from build123d import *

# Parameters (mm, degrees)
BASE_FLANGE1_DEPTH         = 1
SKETCHED_START             = 31
SKETCHED_BEND1_DEPTH       = 178
SKETCHED_BEND1_2_DEPTH     = 128
SKETCHED_BEND1_3_DEPTH     = 178
SKETCHED_BEND1_4_OUTLINE_W = 128
SKETCHED_BEND1_4_OUTLINE_H = 1
SKETCHED_BEND1_4_DEPTH     = 29.234623369
SKETCHED_START_2           = 210.765376631
SKETCHED_BEND1_5_OUTLINE_W = 128
SKETCHED_BEND1_5_OUTLINE_H = 1
SKETCHED_BEND1_5_DEPTH     = 29.234623369
SKETCHED_BEND1_6_DEPTH     = 128
SKETCHED_BEND1_7_OUTLINE_W = 178
SKETCHED_BEND1_7_OUTLINE_H = 1
SKETCHED_BEND1_7_DEPTH     = 29.234623369
SKETCHED_START_3           = 160.765376631
SKETCHED_BEND1_8_OUTLINE_W = 178
SKETCHED_BEND1_8_OUTLINE_H = 1
SKETCHED_BEND1_8_DEPTH     = 29.234623369


# Read off the part's stored shape, not the designer's step: Sketched Bend1
# Sheet-metal steps are written as plain solids
with BuildPart() as part:
    # Sketch1 → Base-Flange1 (new body)
    with BuildSketch(Plane.XY):
        Polygon((0, 209), (31, 209), (31, 240), (159, 240), (159, 209), (190, 209), (190, 31), (159, 31), (159, 0), (31, 0), (31, 31), (0, 31), align=None)
    extrude(amount=-BASE_FLANGE1_DEPTH)

    # Sketched Bend1 outline → Sketched Bend1 (add)
    with BuildSketch(Plane(origin=(0, 0, 0), x_dir=(1, 0, 0), z_dir=(0, 1, 0)).offset(SKETCHED_START)):
        with BuildLine():
            Line((29.234623369, -0.7366), (29.234623369, -29.765376631))
            Line((29.234623369, -29.765376631), (30.234623369, -29.765376631))
            Line((30.234623369, -29.765376631), (30.234623369, -0.7366))
            ThreePointArc((30.234623369, -0.7366), (30.450368514, -0.215745145), (30.971223369, 0))
            Line((30.971223369, 0), (29.398582279, 0))
            ThreePointArc((29.398582279, 0), (29.276108612, -0.359286442), (29.234623369, -0.7366))
        make_face()
        with BuildLine():
            Line((160.601417721, 0), (159.028776631, 0))
            ThreePointArc((159.028776631, 0), (159.549631486, -0.215745145), (159.765376631, -0.7366))
            Line((159.765376631, -0.7366), (159.765376631, -29.765376631))
            Line((159.765376631, -29.765376631), (160.765376631, -29.765376631))
            Line((160.765376631, -29.765376631), (160.765376631, -0.7366))
            ThreePointArc((160.765376631, -0.7366), (160.723891388, -0.359286442), (160.601417721, 0))
        make_face()
    extrude(amount=SKETCHED_BEND1_DEPTH)

    # Sketched Bend1 2 outline → Sketched Bend1 2 (add)
    with BuildSketch(Plane.YZ.offset(SKETCHED_START)):
        with BuildLine():
            Line((209.028776631, 0), (210.601417721, 0))
            ThreePointArc((210.601417721, 0), (210.723891388, 0.359286442), (210.765376631, 0.7366))
            Line((210.765376631, 0.7366), (210.765376631, 29.765376631))
            Line((210.765376631, 29.765376631), (209.765376631, 29.765376631))
            Line((209.765376631, 29.765376631), (209.765376631, 0.7366))
            ThreePointArc((209.765376631, 0.7366), (209.549631486, 0.215745145), (209.028776631, 0))
        make_face()
        with BuildLine():
            ThreePointArc((29.234623369, 0.7366), (29.276108612, 0.359286442), (29.398582279, 0))
            Line((29.398582279, 0), (30.971223369, 0))
            ThreePointArc((30.971223369, 0), (30.450368514, 0.215745145), (30.234623369, 0.7366))
            Line((30.234623369, 0.7366), (30.234623369, 29.765376631))
            Line((30.234623369, 29.765376631), (29.234623369, 29.765376631))
            Line((29.234623369, 29.765376631), (29.234623369, 0.7366))
        make_face()
    extrude(amount=SKETCHED_BEND1_2_DEPTH)

    # Sketched Bend1 3 outline → Sketched Bend1 3 (cut)
    with BuildSketch(Plane(origin=(0, 0, 0), x_dir=(1, 0, 0), z_dir=(0, 1, 0)).offset(SKETCHED_START)):
        with BuildLine():
            Line((0, 0), (29.398582279, 0))
            ThreePointArc((29.398582279, 0), (30.039397205, 0.728828115), (30.971223369, 1))
            Line((30.971223369, 1), (0, 1))
            Line((0, 1), (0, 0))
        make_face()
        with BuildLine():
            Line((190, 1), (159.028776631, 1))
            ThreePointArc((159.028776631, 1), (159.960602795, 0.728828115), (160.601417721, 0))
            Line((160.601417721, 0), (190, 0))
            Line((190, 0), (190, 1))
        make_face()
    extrude(amount=SKETCHED_BEND1_3_DEPTH, mode=Mode.SUBTRACT)

    # Sketched Bend1 4 outline → Sketched Bend1 4 (cut)
    with BuildSketch(Plane(origin=(0, 0, 0), x_dir=(1, 0, 0), z_dir=(0, 1, 0))):
        with Locations((95, 0.5)):
            Rectangle(SKETCHED_BEND1_4_OUTLINE_W, SKETCHED_BEND1_4_OUTLINE_H)
    extrude(amount=SKETCHED_BEND1_4_DEPTH, mode=Mode.SUBTRACT)

    # Sketched Bend1 5 outline → Sketched Bend1 5 (cut)
    with BuildSketch(Plane(origin=(0, 0, 0), x_dir=(1, 0, 0), z_dir=(0, 1, 0)).offset(SKETCHED_START_2)):
        with Locations((95, 0.5)):
            Rectangle(SKETCHED_BEND1_5_OUTLINE_W, SKETCHED_BEND1_5_OUTLINE_H)
    extrude(amount=SKETCHED_BEND1_5_DEPTH, mode=Mode.SUBTRACT)

    # Sketched Bend1 6 outline → Sketched Bend1 6 (cut)
    with BuildSketch(Plane.YZ.offset(SKETCHED_START)):
        with BuildLine():
            ThreePointArc((210.601417721, 0), (209.960602795, -0.728828115), (209.028776631, -1))
            Line((209.028776631, -1), (240, -1))
            Line((240, -1), (240, 0))
            Line((240, 0), (210.601417721, 0))
        make_face()
        with BuildLine():
            Line((0, -1), (30.971223369, -1))
            ThreePointArc((30.971223369, -1), (30.039397205, -0.728828115), (29.398582279, 0))
            Line((29.398582279, 0), (0, 0))
            Line((0, 0), (0, -1))
        make_face()
    extrude(amount=SKETCHED_BEND1_6_DEPTH, mode=Mode.SUBTRACT)

    # Sketched Bend1 7 outline → Sketched Bend1 7 (cut)
    with BuildSketch(Plane.YZ):
        with Locations((120, -0.5)):
            Rectangle(SKETCHED_BEND1_7_OUTLINE_W, SKETCHED_BEND1_7_OUTLINE_H)
    extrude(amount=SKETCHED_BEND1_7_DEPTH, mode=Mode.SUBTRACT)

    # Sketched Bend1 8 outline → Sketched Bend1 8 (cut)
    with BuildSketch(Plane.YZ.offset(SKETCHED_START_3)):
        with Locations((120, -0.5)):
            Rectangle(SKETCHED_BEND1_8_OUTLINE_W, SKETCHED_BEND1_8_OUTLINE_H)
    extrude(amount=SKETCHED_BEND1_8_DEPTH, mode=Mode.SUBTRACT)


solid = part.part
Work out the finished part from the listing and answer in its coordinate system (mm). A direction names the side the tool comes from. Give positions to 0.01 mm unless a question says otherwise; leave off trailing zeros. Loops run counter-clockwise (first coordinate to the right, second up) from the corner with the lowest first, then second, coordinate; pieces in that order, holes last. Notation, with made-up numbers: (55.25, -30.75) -> (69.25, -30.75) arc R22 cw to (69.25, 0.25) -> close; hole circle Ø3 at (7, 0). An arc over 180 degrees is marked (long way). Use a Markdown table: item, result. Add a question column.
1. Flat-ended cylindrical pins translate along their axes: pin 1 Ø0.5 at (x, z) = (30, 19) entering from +Y; pin 2 Ø1.4 at (y, z) = (30.5, 12) entering from +X; pin 3 Ø1.4 at (y, z) = (210, 11.5) entering from -X; pin 4 Ø0.9 at (y, z) = (210, 15.5) entering from +X. Find the tip coordinate at first contact, or state that the pin passes through.
2. Section A-A on z = 19.5 is taken. Determine the outline of the cut face in (x, y), and give its area (3 significant figures).
3. For faces 1 (the flat face through (30.235, 119, 15)), 2 (the flat face through (29.235, 119, 15)), 3 (the flat face through (94, 30.235, 15)), determine the directions among +Z, -Z, +X, -X, +Y, -Y from which every point of the face is accessible in a straight line to the end or side of a thin tool.
4. Determine the mould class of faces 4 (the flat face through (96, 121, 0)), 5 (the flat face through (94, 209.765, 15)), 6 (the flat face through (94, 29.235, 15)), 7 (the flat face through (159.765, 119, 15)) for opening direction Y: released by +Y, released by -Y, zero draft, split by the parting line, or undercut.
5. Section B-B on y = 45 is taken. Determine the outline of the cut face in (x, z), and give its area (3 significant figures).
6. Find the intervals of material crossed by probe 1 along X at (y, z) = (41, 7.5); probe 2 along Y at (x, z) = (131.5, 26); probe 3 along Z at (x, y) = (63, 156.5), in increasing order.
7. Section C-C on x = 84.5 is taken. Determine the outline of the cut face in (y, z), and give its area (3 significant figures).
Results below:
| question | item | result |
|---|---|---|
| 1 | pin 1 | stops at y = 209 |
| 1 | pin 2 | stops at x = 160.77 |
| 1 | pin 3 | stops at x = 31 |
| 1 | pin 4 | stops at x = 159 |
| 2 | outline | (29.23, 31) -> (30.23, 31) -> (30.23, 209) -> (29.23, 209) -> close; (31, 29.23) -> (159, 29.23) -> (159, 30.23) -> (31, 30.23) -> close; (31, 209.77) -> (159, 209.77) -> (159, 210.77) -> (31, 210.77) -> close; (159.77, 31) -> (160.77, 31) -> (160.77, 209) -> (159.77, 209) -> close |
| 2 | area | 612 mm^2 |
| 3 | face 1 | +Z, +Y, -Y |
| 3 | face 2 | +Z, -Z, -X, +Y, -Y |
| 3 | face 3 | +Z, +X, -X |
| 4 | face 4 | undercut |
| 4 | face 5 | undercut |
| 4 | face 6 | released by -Y |
| 4 | face 7 | zero draft |
| 5 | outline | (29.23, 0.74) arc R1.74 ccw to (30.97, -1) -> (159.03, -1) arc R1.74 ccw to (160.77, 0.74) -> (160.77, 29.77) -> (159.77, 29.77) -> (159.77, 0.74) arc R0.74 cw to (159.03, 0) -> (30.97, 0) arc R0.74 cw to (30.23, 0.74) -> (30.23, 29.77) -> (29.23, 29.77) -> close |
| 5 | area | 190 mm^2 |
| 6 | probe 1 | x = 29.23 to 30.23, 159.77 to 160.77 |
| 6 | probe 2 | y = 29.23 to 30.23, 209.77 to 210.77 |
| 6 | probe 3 | z = -1 to 0 |
| 7 | outline | (29.23, 0.74) arc R1.74 ccw to (30.97, -1) -> (209.03, -1) arc R1.74 ccw to (210.77, 0.74) -> (210.77, 29.77) -> (209.77, 29.77) -> (209.77, 0.74) arc R0.74 cw to (209.03, 0) -> (30.97, 0) arc R0.74 cw to (30.23, 0.74) -> (30.23, 29.77) -> (29.23, 29.77) -> close |
| 7 | area | 240 mm^2 |
